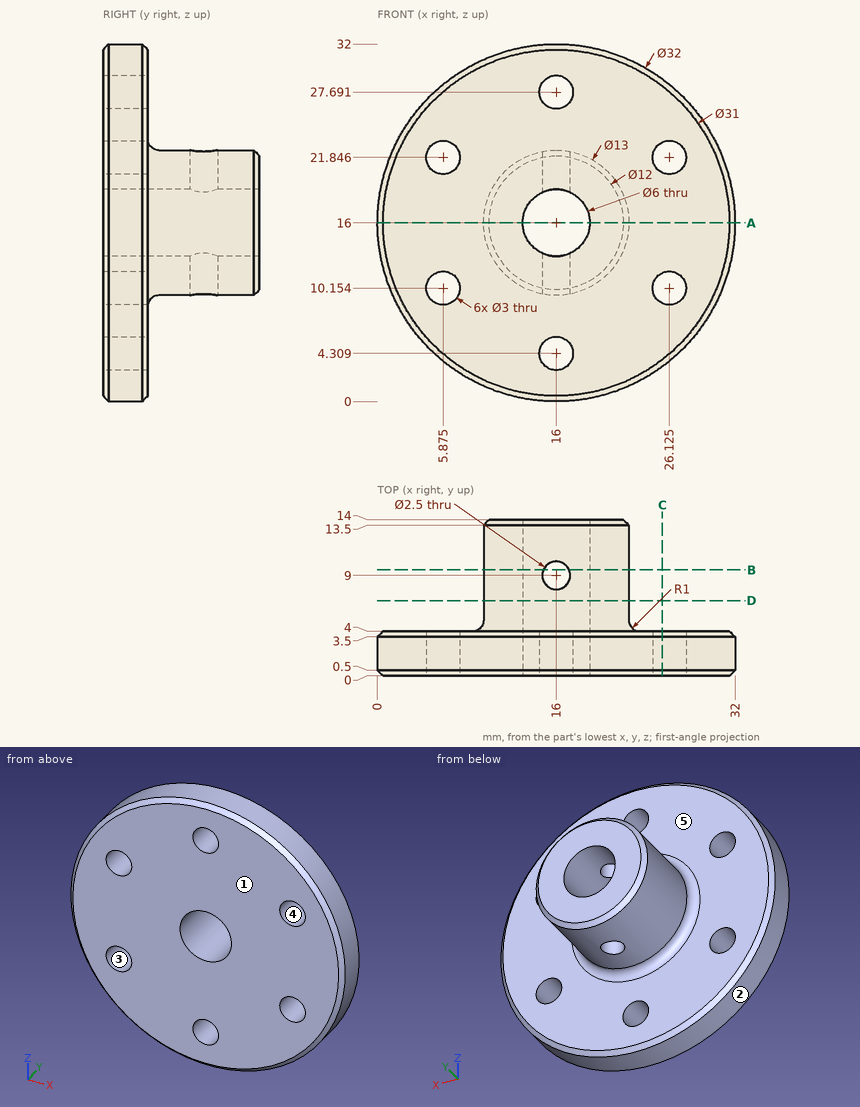
Can you work these out from the drawing? Everything is in mm from the part's minimum corner. A direction names the side the tool comes from. Coordinates: 2 decimals unless noted, no trailing zeros. Order: outer loops, then holes, each group sorted by start corner. A loop starts at its lowest first (then second) coordinate and runs counter-clockwise, first axis right, second up. Notation, with made-up numbers: (-13.5, 16.5) -> (28.5, 16.5) arc R28 cw to (28.5, 44.5) -> close; hole circle Ø11 at (-1.75, 23.25). An arc over 180 degrees is marked (long way). Return JSON: item names as keys, results as strings.
1) If we section it at C-C on x = 25.5: State how many separate pieces and enclosed holes the cut face has.
Conclusion:
{"separate pieces": "3", "enclosed holes": "0"}
2) If we section it at D-D on y = 6.75: List the corners of the cut face in (x, z) for me.
Conclusion:
{"outline": "circle Ø13 at (16, 16); hole circle Ø6 at (16, 16)"}
3) Thinking about a two-plate mould opening in Z: for the marked faces 1, 2 and 3, which applies, +Z half, -Z half, draft (parallel to the pull), parting line (faces both ways), or undercut?
Conclusion:
{"face 1": "draft", "face 2": "parting line", "face 3": "undercut"}
4) If I drill on probe 1 along Y at (x, z) = (14, 5.5); probe 2 along X at (y, z) = (8, 16); probe 3 along Z at (x, y) = (5, 3.25) (1 decimal), over which ranges is the centre line in solid material (lowest first)?
Conclusion:
{"probe 1": "y = 0 to 4", "probe 2": "x = 9.5 to 13, 19 to 22.5", "probe 3": "z = 4.4 to 8.9, 11.4 to 20.6, 23.1 to 27.6"}
5) If we section it at A-A on z = 16: List the corners of the cut face in (x, y) for me.
Conclusion:
{"outline": "(0, 0.5) -> (0.5, 0) -> (13, 0) -> (13, 14) -> (10, 14) -> (9.5, 13.5) -> (9.5, 5) arc R1 cw to (8.5, 4) -> (0.5, 4) -> (0, 3.5) -> close; (19, 0) -> (31.5, 0) -> (32, 0.5) -> (32, 3.5) -> (31.5, 4) -> (23.5, 4) arc R1 cw to (22.5, 5) -> (22.5, 13.5) -> (22, 14) -> (19, 14) -> close"}
6) On a 3-axis mill with a long thin cutter (end or side, diameter ignored), from which of +Z, -Z, +X, -X, +Y, -Y can I reach the whole of each face in a straight line? I mean the marked faces 4 and 5. Say none if no direction works.
Conclusion:
{"face 4": "+Y, -Y", "face 5": "+Y"}
7) I'm going to push flat-ended pins straight in: P1, Ø1, axis at y = 4, z = 27.5, coming from the +X side (1 decimal); P2, Ø1, axis at x = 19.5, y = 7.5, coming from the +Z side; P3, Ø1, axis at y = 3, z = 14.5, coming from the +X side. Where does each tip first touch, or does it pass through?
Conclusion:
{"P1": "stops at x = 27.3", "P2": "stops at z = 21.77", "P3": "stops at x = 31.97"}
8) If we section it at B-B on y = 9.5: List the corners of the cut face in (x, z) for me (1 decimal).
Conclusion:
{"outline": "(14.9, 9.6) -> (14.9, 13.2) arc R3 cw to (14.9, 18.8) -> (14.9, 22.4) arc R6.5 ccw to start; (17.1, 9.6) arc R6.5 ccw to (17.1, 22.4) -> (17.1, 18.8) arc R3 cw to (17.1, 13.2) -> close"}
